Verification items for the finished model (mm, model axes). A direction names the side the tool comes from. Round coordinates to 2 decimals unless told otherwise and drop trailing zeros. Write each loop counter-clockwise with the first axis right and the second up, starting at its lowest first coordinate (ties: lowest second). Pieces come first, ordered by that corner, then holes. Notation, with made-up numbers: (31.25, 79.25) -> (70.25, 79.25) arc R11 ccw to (70.25, 94.25) -> close; hole circle Ø9 at (28.5, 19). An arc over 180 degrees is marked (long way). Use CSV: the item, a comma, the result in double quotes.
```python
from build123d import *

# Parameters (mm, degrees)
CENTER_BODY_DEPTH               = 10
SKETCH1_3_R                     = 1.6
SKETCH1_3_R_2                   = 1.6000000000000003
CONNECTOR_BODY_DEPTH            = 5
MECH_LOCK_RIGHT_DEPTH           = 5
DULLING_FILLET_GENERAL_R        = 0.5
ELEPHANTSFOOT_COMPENSATION_SIZE = 0.16
DULLING_FILLET_RIGHT_R          = 0.5


with BuildPart() as part:
    # complete_sketch → center_body (new body)
    with BuildSketch(Plane(origin=(0, 0, 0), x_dir=(1, 0, 0), z_dir=(0, 1, 0))):
        Polygon((-5, 47), (-5, 4.195498155886381), (5, 5.958767962971076), (5, 47), align=None)
    extrude(amount=CENTER_BODY_DEPTH)

    # Sketch1_3 → connector_body (add)
    # profile 1 of 2: a face of its own
    with BuildSketch(Plane(origin=(0, 0, 0), x_dir=(1, 0, 0), z_dir=(0, 1, 0))):
        with BuildLine():
            Line((-5, 4.195498155886381), (-5, 0))
            ThreePointArc((-5, 0), (-3.1e-16, -5), (5, -6.1e-16))
            Line((5, 0), (5, 5.958767962971076))
            Line((5, 5.958767962971076), (-5, 4.195498155886381))
        make_face()
        with Locations(Location((0, 0, 0), (0, 0, 270))):
            Circle(SKETCH1_3_R, mode=Mode.SUBTRACT)
    # profile 2 of 2: a face of its own
    with BuildSketch(Plane(origin=(0, 0, 0), x_dir=(1, 0, 0), z_dir=(0, 1, 0))):
        with BuildLine():
            Line((-5, 52.70871215252208), (-5, 47))
            Line((-5, 47), (5, 47))
            Line((5, 47), (5, 52.70871215252208))
            Line((5, 52.70871215252208), (5, 55))
            ThreePointArc((5, 55), (-1.4e-16, 60), (-5, 55))
            Line((-5, 55), (-5, 52.70871215252208))
        make_face()
        with Locations(Location((0, 55, 0), (0, 0, 270))):
            Circle(SKETCH1_3_R_2, mode=Mode.SUBTRACT)
    extrude(amount=CONNECTOR_BODY_DEPTH)

    # Sketch2 → mech_lock_right (add)
    with BuildSketch(Plane(origin=(0, 5, 0), x_dir=(1, 0, 0), z_dir=(0, 1, 0))):
        with BuildLine():
            Line((5, 47), (-5, 47))
            Line((-5, 47), (-5, 55))
            ThreePointArc((-5, 55), (-3.5355339059327315, 51.46446609406727), (0, 50))
            ThreePointArc((0, 50), (2.7235158716690253, 48.87252645278171), (5, 47))
        make_face()
    extrude(amount=MECH_LOCK_RIGHT_DEPTH)

    # dulling_fillet_general
    dulling_fillet_general_edges = [part.edges().sort_by_distance(p)[0] for p in [
        (5, 7.5, -5.958767962971076),
        (-5, 7.5, -4.195498155886381),
    ]]
    fillet(dulling_fillet_general_edges, radius=DULLING_FILLET_GENERAL_R)

    # elephantsfoot_compensation
    elephantsfoot_compensation_edges = [part.edges().sort_by_distance(p)[0] for p in [
        (1.4e-16, 0, 5),
        (4.9e-16, 0, -1.6),
        (-1.4e-16, 0, -60),
        (4.9e-16, 0, -56.6),
        (5, 0, -27.5),
        (-5, 0, -27.5),
    ]]
    chamfer(elephantsfoot_compensation_edges, length=ELEPHANTSFOOT_COMPENSATION_SIZE)

    # dulling_fillet_right
    dulling_fillet_right_edges = [part.edges().sort_by_distance(p)[0] for p in [
        (-4.999999999999998, 7.5, -55),
    ]]
    fillet(dulling_fillet_right_edges, radius=DULLING_FILLET_RIGHT_R)


solid = part.part
```
Q1. Access from +Z, -Z, +X, -X, +Y, -Y to the whole of each face (thin tool, end or side, straight path). Record for faces 1 (the cylindrical face through (2.688, 7.465, -48.894)), 2 (the flat face through (-5, 5, -27)), 3 (the flat face through (0.02, 7.46, -5.08)).
Filled in:
face 1,"-Z, +X, +Y"
face 2,"+Z, -Z, -X, +Y, -Y"
face 3,"+Z, +X, +Y"
Q2. Section check B-B (y = 9). Record the cut outline in (x, z).
Filled in:
outline,"(-5, -51.84) arc R0.5 ccw to (-4.09, -52.13) arc R5 cw to (0, -50) arc R10 ccw to (5, -47) -> (5, -6.38) arc R0.5 ccw to (4.59, -5.89) -> (-4.41, -4.3) arc R0.5 ccw to (-5, -4.79) -> close"
Q3. Go/stop test with flat-tipped pins: P1, Ø2, axis at x = -1, y = 8, coming from the -Z side; P2, Ø2, axis at x = -1, y = 6.5, coming from the +Z side; P3, Ø3, axis at x = 2, z = -53, coming from the +Y side; P4, Ø1.9, axis at x = 0, z = -55, coming from the -Y side. Record where each tip stops, or that it passes through.
Filled in:
P1,"z = -50.42"
P2,"z = -4.72"
P3,"y = 5"
P4,"through"
Q4. Mould release check, pull along X, two halves, no side actions. Record for faces 4 (the cylindrical face through (0, 3, 5)), 5 (the cylindrical face through (-0.97, 2.55, -1.27)), 6 (the cylindrical face through (-2.335, 7.465, -50.579)): released by +X, released by -X, zero draft, split by the parting line, or undercut.
Filled in:
face 4,"split by the parting line"
face 5,"undercut"
face 6,"released by +X"
Q5. Section check A-A (y = 2). Record the cut outline in (x, z), plus the area to 3 significant figures.
Filled in:
outline,"(-5, -55) arc R5 ccw to (5, -55) -> (5, 0) arc R5 ccw to (-5, 0) -> close; hole circle Ø3.2 at (0, -55); hole circle Ø3.2 at (0, 0)"
area,"612 mm²"
Q6. Material ranges on L1, parallel to Z at x = -1.25, y = 3.5; L2, parallel to X at y = 2.15, z = -55; L3, parallel to X at y = 2, z = -1, recorded low to high.
Filled in:
L1,"-59.84 to -56, -54 to -1, 1 to 4.84"
L2,"-5 to -1.6, 1.6 to 5"
L3,"-5 to -1.25, 1.25 to 5"
